Input: part model. Units: mm. Frame: model coordinates. A direction names the side the tool comes from. Coordinates: 2 decimals unless noted, no trailing zeros. Write each loop counter-clockwise with the first axis right and the second up, starting at its lowest first coordinate (ties: lowest second). Pieces come first, ordered by that corner, then holes. Notation, with made-up numbers: (75, 21) -> (132, 21) arc R23 ccw to (132, 53) -> close; hole circle Ø9 at (19.5, -3). An arc over 180 degrees is marked (long way). Use one line per item in the form item = value. Start each with the question number.
(1) Cut plane A-A on y = 20.5. Return the cut outline in (x, z), plus the area to 3 significant figures.
(2) Cut plane B-B on x = 5.5. Return the cut outline in (y, z), plus the area to 3 significant figures.
(3) First-contact query: pin 1 (1.5 mm diameter, centred on x = 5.5, z = 8, fed in from +Y); pin 2 (3 mm diameter, centred on x = 8, z = 3.5, fed in from +Y); pin 3 (5 mm diameter, centred on x = 8.5, z = 5, fed in from +Y). Flat tips, straight axial feed; report the tip coordinate or a pass-through.
(4) Cut plane D-D on x = 8. Return the cut outline in (y, z) (3 decimals), plus the area to 3 significant figures.
(5) Ray query, line 1 along X through (y, z) = (3.5, 3.5); line 2 along X through (y, z) = (0.75, 5) (3 decimals); line 3 along Y through (x, z) = (6.5, 9). Return the intervals inside material, ascending.
(6) Pull-direction query (X, two-part tool) for faces 1 (the face through (10.784, 1.965, 3.422)), 2 (the face through (0, 18, 5)), 3 (the face through (2.8, 16.8, 0)); classes: released by +X, released by -X, zero draft, split by the parting line, or undercut.
(7) Set-up query: faces 4 (the face through (5.216, 1.965, 6.578)), 5 (the face through (16, 18, 5)), 6 (the face through (9.098, 0.456, 3.802)). Return all of +Z, -Z, +X, -X, +Y, -Y with unobstructed straight access to the full face (end or side cutting, diameter ignored); none if empty.
(8) Cut plane C-C on z = 7.5. Return the cut outline in (x, y).
```python
from build123d import *

# Parameters (mm, degrees)
SKETCH1_W           = 10
SKETCH1_H           = 34
BOSS_EXTRUDE1_DEPTH = 3
SKETCH2_W           = 10
SKETCH2_H           = 3
BOSS_EXTRUDE2_DEPTH = 3
SKETCH2_4_W         = 10
SKETCH2_4_H         = 3
BOSS_EXTRUDE3_DEPTH = 10
SKETCH6_R           = 1.625
CUT_EXTRUDE3_DEPTH  = 2.1
SKETCH6_3_R         = 1.625
CUT_EXTRUDE4_DEPTH  = 38.056556836
SKETCH5_R           = 1.625
CUT_EXTRUDE5_DEPTH  = 2.1
SKETCH5_4_R         = 1.625
CUT_EXTRUDE6_DEPTH  = 38.268461324


with BuildPart() as part:
    # Sketch1 → Boss-Extrude1 (new body)
    with BuildSketch(Plane(origin=(0, 0, 0), x_dir=(0, 0, -1), z_dir=(1, 0, 0))):
        with Locations((-5, 17)):
            Rectangle(SKETCH1_W, SKETCH1_H)
        Polygon((-10, 35.139356083), (0, 34), (-10, 34), align=None)
    extrude(amount=BOSS_EXTRUDE1_DEPTH)



with BuildPart() as body_2:
    # Sketch2 → Boss-Extrude2 (new body)
    with BuildSketch(Plane(origin=(13, 0, 0), x_dir=(0, 0, -1), z_dir=(1, 0, 0))):
        with Locations((-5, 1.5)):
            Rectangle(SKETCH2_W, SKETCH2_H)
        Polygon((-10, 3), (0, 3), (0, 30.980590802), (-10, 32.119946885), align=None)
        Polygon((-10, 32.119946885), (0, 30.980590802), (0, 34), (-10, 34), align=None)
        Polygon((-10, 34), (0, 34), (-10, 35.139356083), align=None)
    extrude(amount=BOSS_EXTRUDE2_DEPTH)


with BuildPart() as part_1:
    add(part.part)

    add(body_2.part)  # Boss-Extrude3 merges body 2
    # Sketch2<4> → Boss-Extrude3 (add)
    with BuildSketch(Plane(origin=(13, 0, 0), x_dir=(0, 0, -1), z_dir=(1, 0, 0))):
        with Locations((-5, 1.5)):
            Rectangle(SKETCH2_4_W, SKETCH2_4_H)
        Polygon((-10, 32.119946885), (0, 30.980590802), (0, 34), (-10, 34), align=None)
        Polygon((0, 34), (-10, 34), (-10, 35.139356083), align=None)
    extrude(amount=-BOSS_EXTRUDE3_DEPTH)

    # Sketch6 → Cut-Extrude3 (cut)
    # profile 1 of 2: a face of its own
    with BuildSketch(Plane(origin=(0, 30.583575534, -3.484558283), x_dir=(1, 0, 0), z_dir=(0, -0.9935718556765885, 0.11320321376789935))):
        Polygon((4.304958277, 8.539451107), (6.152479139, 5.339451107), (9.847520861, 5.339451107), (11.695041723, 8.539451107), (9.847520861, 11.739451107), (6.152479139, 11.739451107), align=None)
        with Locations((8, 8.539451107)):
            Circle(SKETCH6_R, mode=Mode.SUBTRACT)
    # profile 2 of 2: a face of its own
    with BuildSketch(Plane(origin=(0, 30.583575534, -3.484558283), x_dir=(1, 0, 0), z_dir=(0, -0.9935718556765885, 0.11320321376789935))):
        with Locations((8, 8.539451107)):
            Circle(SKETCH6_R)
    extrude(amount=-CUT_EXTRUDE3_DEPTH, mode=Mode.SUBTRACT)

    # Sketch6<3> → Cut-Extrude4 (cut, through all)
    with BuildSketch(Plane(origin=(0, 30.583575534, -3.484558283), x_dir=(1, 0, 0), z_dir=(0, -0.9935718556765885, 0.11320321376789935))):
        with Locations(Location((8, 8.539451107, 0), (0, 0, 270))):
            Circle(SKETCH6_3_R)
    extrude(amount=-CUT_EXTRUDE4_DEPTH, mode=Mode.SUBTRACT)

    # Sketch5 → Cut-Extrude5 (cut)
    with BuildSketch(Plane(origin=(0, 3, 0), x_dir=(1, 0, 0), z_dir=(0, 1, 0))):
        Polygon((6.152479139, -1.8), (4.304958277, -5), (6.152479139, -8.2), (9.847520861, -8.2), (11.695041723, -5), (9.847520861, -1.8), align=None)
        with Locations(Location((8, -5, 0), (0, 0, 270))):
            Circle(SKETCH5_R, mode=Mode.SUBTRACT)
    extrude(amount=-CUT_EXTRUDE5_DEPTH, mode=Mode.SUBTRACT)

    # Sketch5<4> → Cut-Extrude6 (cut, through all)
    with BuildSketch(Plane(origin=(0, 3, 0), x_dir=(1, 0, 0), z_dir=(0, 1, 0))):
        with Locations(Location((8, -5, 0), (0, 0, 270))):
            Circle(SKETCH5_4_R)
    extrude(amount=-CUT_EXTRUDE6_DEPTH, mode=Mode.SUBTRACT)


solid = part_1.part
```
Values:
q1.outline = (0, 0) -> (3, 0) -> (3, 10) -> (0, 10) -> close; (13, 0) -> (16, 0) -> (16, 10) -> (13, 10) -> close
q1.area = 60.0 mm2
q2.outline = (0, 0) -> (3, 0) -> (3, 2.93) -> (0.9, 2.93) -> (0.9, 7.07) -> (3, 7.07) -> (3, 10) -> (0, 10) -> close; (30.98, 0) -> (34, 0) -> (35.14, 10) -> (32.12, 10) -> (31.78, 7.06) -> (33.87, 6.82) -> (33.4, 2.71) -> (31.32, 2.94) -> close
q2.area = 42.8 mm2
q3.pin_1 = 35
q3.pin_2 = 34.45
q3.pin_3 = 34.85
q4.outline = (0, 0) -> (3, 0) -> (3, 1.8) -> (0.9, 1.8) -> (0.9, 3.375) -> (0, 3.375) -> close; (0, 6.625) -> (0.9, 6.625) -> (0.9, 8.2) -> (3, 8.2) -> (3, 10) -> (0, 10) -> close; (30.981, 0) -> (34, 0) -> (34.347, 3.046) -> (33.453, 3.148) -> (33.275, 1.583) -> (31.188, 1.821) -> close; (31.913, 8.179) -> (33.999, 7.942) -> (33.821, 6.377) -> (34.715, 6.275) -> (35.139, 10) -> (32.12, 10) -> close
q4.area = 27.5 mm2
q5.line_1 = 0 to 3, 13 to 16
q5.line_2 = 0 to 6.375, 9.625 to 16
q5.line_3 = 0 to 3, 32.01 to 35.03
q6.face_1 = undercut
q6.face_2 = released by -X
q6.face_3 = zero draft
q7.face_4 = none
q7.face_5 = +Z, -Z, +X, +Y, -Y
q7.face_6 = -Y
q8.outline = (0, 0) -> (16, 0) -> (16, 34.85) -> (0, 34.85) -> close; hole (3, 3) -> (5.75, 3) -> (5.75, 0.9) -> (10.25, 0.9) -> (10.25, 3) -> (13, 3) -> (13, 31.84) -> (10.24, 31.84) -> (10.1, 33.95) -> (5.9, 33.95) -> (5.76, 31.84) -> (3, 31.84) -> close
